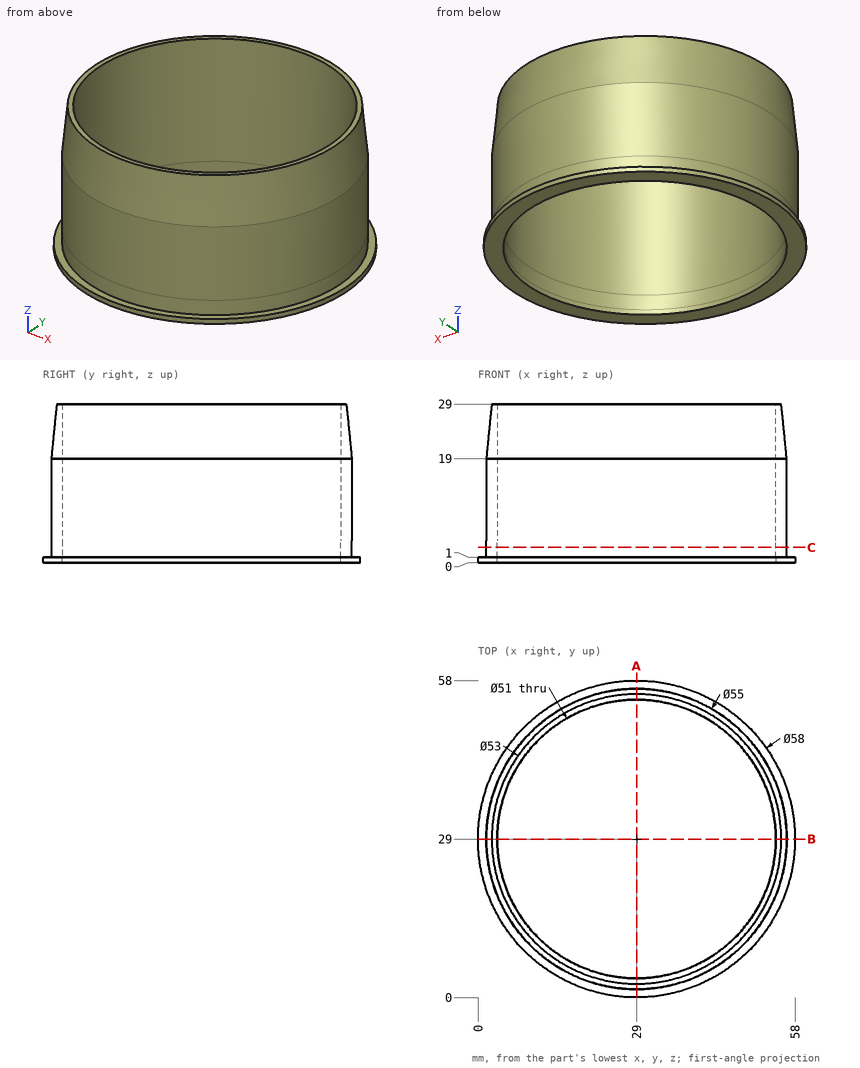
Source: three-view drawing plus pictorial views. Frame: mm from the lowest corner of the part. Give positions to 0.01 mm unless a question says otherwise; leave off trailing zeros. Write each loop counter-clockwise with the first axis right and the second up, starting at its lowest first coordinate (ties: lowest second). Pieces come first, ordered by that corner, then holes. Notation, with made-up numbers: (56, 41) -> (61, 41) arc R18 cw to (61, 60) -> close; hole circle Ø8 at (76.25, 21.25). An arc over 180 degrees is marked (long way). Write item = value, one per line.
Q1. Cut plane A-A on x = 29. Return loops of the section in (y, z), then the cut area to 3 significant figures.
Here are the results:
outline = (0, 0) -> (3.5, 0) -> (3.5, 29) -> (2.5, 29) -> (1.5, 19) -> (1.5, 1) -> (0, 1) -> close; (54.5, 0) -> (58, 0) -> (58, 1) -> (56.5, 1) -> (56.5, 19) -> (55.5, 29) -> (54.5, 29) -> close
area = 109 mm²
Q2. Line query: line 1 (X direction, y = 29, z = 17); line 2 (X direction, y = 29, z = 0.8). Output: solid intervals per line, ascending. Write a range as from..to.
Here are the results:
line_1 = 1.5..3.5, 54.5..56.5
line_2 = 0..3.5, 54.5..58
Q3. Cut plane C-C on z = 2.75. Return loops of the section in (x, y), then the cut area to 3 significant figures.
Here are the results:
outline = circle Ø55 at (29, 29); hole circle Ø51 at (29, 29)
area = 333 mm²
Q4. First-contact query: pin 1 (4 mm diameter, centred on y = 16.5, z = 20.5, fed in from -X); pin 2 (2 mm diameter, centred on x = 6.5, z = 12, fed in from -Y); pin 3 (8 mm diameter, centred on x = 26.5, z = 7.5, fed in from -Y); pin 4 (17.5 mm diameter, centred on x = 42.5, y = 33.5, fed in from +Z). Flat tips, straight axial feed; report the tip coordinate or a pass-through.
Here are the results:
pin_1 = 3.72
pin_2 = 11.85
pin_3 = 1.5
pin_4 = through
